The model under review builds one solid part; all positions refer to its coordinate system, in mm. Face numbers are marked on the shaded views. A direction names the side the tool comes from. Round coordinates to 2 decimals unless told otherwise and drop trailing zeros. Write each loop counter-clockwise with the first axis right and the second up, starting at its lowest first coordinate (ties: lowest second). Pieces come first, ordered by that corner, then holes. Notation, with made-up numbers: (8.5, -28) - (61.5, -28) arc R11 ccw to (61.5, -17) - close; hole circle Ø7 at (34.25, 35.5). An arc over 180 degrees is marked (long way). Write each question's results on one line, items separated by ' | '.
```python
from build123d import *

# Parameters (mm, degrees)
F1_DEPTH = 50


with BuildPart() as f1:
    # F0 (on Front) → F1 (new body)
    with BuildSketch(Plane.XZ):
        Polygon((25, -25), (50, -25), (50, 17.929452), (27.833339, 2.565201), (1.583336, 7.62179), (-17.277775, 5.871432), (-39.638888, 1.093402), (-56.633994, -7.194445), (-69.316667, -7.194445), (-80, -25), (-50, -25), align=None)
        with BuildLine():
            ThreePointArc((-50, -18.25), (-50.883883, -16.116117), (-48.75, -17))
            ThreePointArc((-48.75, -17), (-49.116117, -17.883883), (-50, -18.25))
        make_face(mode=Mode.SUBTRACT)
        with BuildLine():
            ThreePointArc((25, -18.25), (24.116117, -16.116117), (26.25, -17))
            ThreePointArc((26.25, -17), (25.883883, -17.883883), (25, -18.25))
        make_face(mode=Mode.SUBTRACT)
    extrude(amount=F1_DEPTH)


solid = f1.part
```
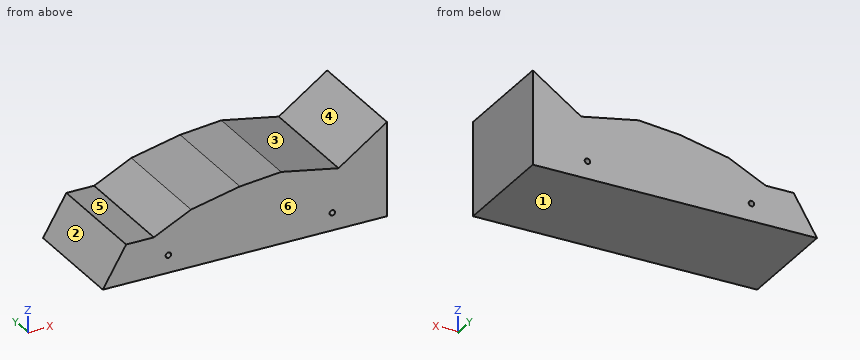
Q1. We need section A-A (y = -43). State the section outline as (x, z) points, plus the area to 3 significant figures.
Evaluation:
outline: (-80, -25) - (50, -25) - (50, 17.93) - (27.83, 2.57) - (1.58, 7.62) - (-17.28, 5.87) - (-39.64, 1.09) - (-56.63, -7.19) - (-69.32, -7.19) - close; hole (-50, -18.25) arc R1.25 ccw to (-48.75, -17) arc R1.25 ccw (long way) to start; hole (25, -18.25) arc R1.25 ccw to (26.25, -17) arc R1.25 ccw (long way) to start | area: 3,490 mm^2
Q2. For probe 1 along X at (y, z) = (-32, -17); probe 2 along X at (y, z) = (-15.5, -16); probe 3 along Z at (x, y) = (25, -26.5), list the stretches that pass through material, from the lowest coordinate up.
Evaluation:
probe 1: x = -75.2 to -51.25, -48.75 to 23.75, 26.25 to 50 | probe 2: x = -74.6 to -50.75, -49.25 to 24.25, 25.75 to 50 | probe 3: z = -25 to -18.25, -15.75 to 3.11
Q3. We need section B-B (x = -58). State the section outline as (y, z) points, plus the area to 3 significant figures.
Evaluation:
outline: (-50, -25) - (0, -25) - (0, -7.19) - (-50, -7.19) - close | area: 890 mm^2
Q4. Insertion check: P1, Ø14, axis at x = -61.5, y = -32.5, coming from the +Z side. The pin has a flat end and moves straight along its axis. Give the tip position at first contact, or say it passes through.
Evaluation:
P1: stops at z = -6.15
Q5. Tool access review of the marked faces 4, 5 and 6: name each direction out of +Z, -Z, +X, -X, +Y, -Y from which nothing blocks a thin tool from reaching the whole face with its end or side.
Evaluation:
face 4: +Z, +Y, -Y | face 5: +Z, -X, +Y, -Y | face 6: +Z, -Z, +X, -X, -Y
Q6. We need section C-C (z = -9.5). State the section outline as (x, y) points, plus the area to 4 significant figures.
Evaluation:
outline: (-70.7, -50) - (50, -50) - (50, 0) - (-70.7, 0) - close | area: 6,035 mm^2
Q7. The part is to be moulded in two halves that separate along X. For the marked faces 1, 2 and 3, say which applies: released by +X, released by -X, zero draft, split by the parting line, or undercut.
Evaluation:
face 1: zero draft | face 2: released by -X | face 3: undercut
